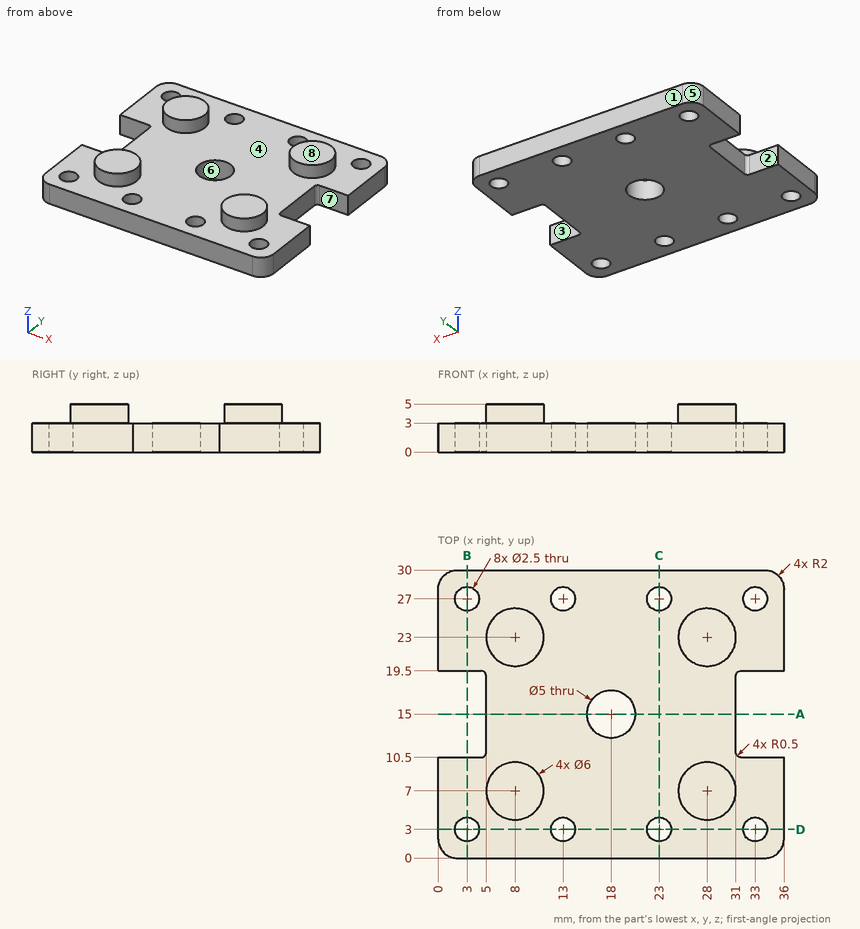
Design review of the part shown in the three views and the two pictorial views. Dimensions are in mm from the part's minimum x, y and z. A direction names the side the tool comes from. Round coordinates to 2 decimals unless told otherwise and drop trailing zeros. Write each loop counter-clockwise with the first axis right and the second up, starting at its lowest first coordinate (ties: lowest second). Pieces come first, ordered by that corner, then holes. Notation, with made-up numbers: M 12.5,47 L 48.5,47 A14 cw 48.5,60 Z; hole C 16.25,49 d10. An arc over 180 degrees is marked long. Use a Markdown table: item, result. Add a question column.
Q1. To check wall thickness, follow line 1 (Y direction, x = 33, z = 2.2); line 2 (Y direction, x = 23, z = 0.6); line 3 (Y direction, x = 2.5, z = 0.7). State the ranges of each line that lie inside material, in increasing order.
Q2. The part is to be moulded in two halves that separate along Y. For the marked faces 5, 6, 7 and 8, say which applies: pulls with the +Y half, pulls with the -Y half, needs draft (parallel to the pull), parting line crosses it, or undercut.
Q3. We need section C-C, the plane x = 23. State the section outline as (y, z) points.
Q4. We need section A-A, the plane y = 15. State the section outline as (x, z) points, plus the area to 3 significant figures.
Q5. We need section D-D, the plane y = 3. State the section outline as (x, z) points.
Q6. We need section B-B, the plane x = 3. State the section outline as (y, z) points, plus the area to 3 significant figures.
Q7. Insertion check: pin 1 (3 mm diameter, centred on x = 13, y = 3, fed in from +Z); pin 2 (0.9 mm diameter, centred on x = 1, z = 1.5, fed in from -Y); pin 3 (2.5 mm diameter, centred on y = 13.5, z = 1, fed in from -X). Each pin has a flat end and moves straight along its axis. Give the tip position at first contact, or say it passes through.
Q8. Machinability: for the marked faces 1, 2, 3 and 4, which of the approach directions +Z, -Z, +X, -X, +Y, -Y give a long, thin tool a straight path to every point of the face, cutting with its end or side? Answer none if there is none.
Findings below:
| question | item | result |
|---|---|---|
| 1 | line 1 | y = 0 to 1.75, 4.25 to 10.5, 19.5 to 25.75, 28.25 to 30 |
| 1 | line 2 | y = 0 to 1.75, 4.25 to 25.75, 28.25 to 30 |
| 1 | line 3 | y = 0 to 1.85, 4.15 to 10.5, 19.5 to 25.85, 28.15 to 30 |
| 2 | face 5 | pulls with the +Y half |
| 2 | face 6 | undercut |
| 2 | face 7 | undercut |
| 2 | face 8 | needs draft |
| 3 | outline | M 0,0 L 1.75,0 L 1.75,3 L 0,3 Z; M 4.25,0 L 25.75,0 L 25.75,3 L 4.25,3 Z; M 28.25,0 L 30,0 L 30,3 L 28.25,3 Z |
| 4 | outline | M 5,0 L 15.5,0 L 15.5,3 L 5,3 Z; M 20.5,0 L 31,0 L 31,3 L 20.5,3 Z |
| 4 | area | 63.0 mm² |
| 5 | outline | M 0,0 L 1.75,0 L 1.75,3 L 0,3 Z; M 4.25,0 L 11.75,0 L 11.75,3 L 4.25,3 Z; M 14.25,0 L 21.75,0 L 21.75,3 L 14.25,3 Z; M 24.25,0 L 31.75,0 L 31.75,3 L 24.25,3 Z; M 34.25,0 L 36,0 L 36,3 L 34.25,3 Z |
| 6 | outline | M 0,0 L 1.75,0 L 1.75,3 L 0,3 Z; M 4.25,0 L 10.5,0 L 10.5,3 L 4.25,3 Z; M 19.5,0 L 25.75,0 L 25.75,3 L 19.5,3 Z; M 28.25,0 L 30,0 L 30,3 L 28.25,3 Z |
| 6 | area | 48.0 mm² |
| 7 | pin 1 | stops at z = 3 |
| 7 | pin 2 | stops at y = 0.08 |
| 7 | pin 3 | stops at x = 5 |
| 8 | face 1 | +Z, -Z, +X, -X, +Y |
| 8 | face 2 | +Z, -Z, -X |
| 8 | face 3 | +Z, -Z, +X |
| 8 | face 4 | +Z |
